CAD build for the part. Positions are in the model's coordinates, mm. A direction names the side the tool comes from. Round coordinates to 2 decimals unless told otherwise and drop trailing zeros. Write each loop counter-clockwise with the first axis right and the second up, starting at its lowest first coordinate (ties: lowest second). Pieces come first, ordered by that corner, then holes. Notation, with made-up numbers: (81.25, 22) -> (106.25, 22) arc R22 cw to (106.25, 59) -> close; hole circle Ø10 at (7.25, 16.5). An arc over 180 degrees is marked (long way). Answer in a Markdown table with one row per item. Add a question column.
Autodesk Inventor part; units mm, degrees
ref_plane "YZ Plane" through (0, 0, 0) normal (1, 0, 0) x (0, 1, 0)
ref_plane "XZ Plane" through (0, 0, 0) normal (0, 1, 0) x (-1, 0, 0)
ref_plane "XY Plane" through (0, 0, 0) normal (0, 0, 1) x (1, 0, 0)
sketch "スケッチ1" plane through (0, 0, 0) normal (0, 0, 1) x (1, 0, 0)
  line L0 (0, 0) -> (32, 0)
  line L1 (32, 0) -> (32, 32)
  line L2 (32, 32) -> (0, 32)
  line L3 (0, 32) -> (0, 0)
  dimension "d0" = 32
  dimension "d1" = 32
extrude "押し出し1" add sketch "スケッチ1" along normal blind 1.6
sketch "スケッチ2" plane through (0, 0, 1.6) normal (0, 0, 1) x (1, 0, 0)
  line L0 (0, 0) -> (32, 0)
  line L1 (32, 0) -> (32, 32)
  line L2 (32, 32) -> (0, 32)
  line L3 (0, 32) -> (0, 0)
  line L4 (30, 2) -> (2, 2)
  line L5 (2, 2) -> (2, 30)
  line L6 (2, 30) -> (30, 30)
  line L7 (30, 30) -> (30, 2)
  dimension "d4" = 28
hole "穴1" at (30, 30, 1.6) at (30, 2, 1.6) at (2, 2, 1.6) at (2, 30, 1.6) direction (0, 0, -1) diameter 2 end through all
sketch "スケッチ3" plane through (0, 0, 1.6) normal (0, 0, 1) x (1, 0, 0)
  line L0 (5.5, 26.5) -> (26.5, 26.5)
  line L1 (26.5, 26.5) -> (26.5, 5.5)
  line L2 (26.5, 5.5) -> (5.5, 5.5)
  line L3 (5.5, 5.5) -> (5.5, 26.5)
  circle A0 centre (2, 2) radius 1
  circle A1 centre (30, 30) radius 1
  circle A2 centre (30, 2) radius 1
  circle A3 centre (2, 30) radius 1
  line L4 (0, 0) -> (32, 0)
  line L5 (32, 0) -> (32, 32)
  line L6 (32, 32) -> (0, 32)
  line L7 (0, 32) -> (0, 0)
  line L8 (16, 26.5) -> (16, 32)
  line L9 (32, 32) -> (0, 32)
  line L10 (5.5, 16) -> (0, 16)
  line L11 (0, 32) -> (0, 0)
  dimension "d12" = 21
  dimension "d13" = 21
extrude "押し出し2" add sketch "スケッチ3" along normal blind 6.3 contours L0 L1 L2 L3
sketch "スケッチ4" plane through (0, 0, 7.9) normal (0, 0, 1) x (1, 0, 0)
  line L0 (5.5, 26.5) -> (5.5, 5.5)
  line L1 (5.5, 5.5) -> (26.5, 5.5)
  line L2 (26.5, 5.5) -> (26.5, 26.5)
  line L3 (26.5, 26.5) -> (5.5, 26.5)
  line L4 (5.5, 26.5) -> (26.5, 26.5)
  line L5 (16, 26.5) -> (16, 5.5)
  line L6 (5.5, 5.5) -> (26.5, 5.5)
  circle A0 centre (16, 16) radius 9.5
  point P0 (0, 0)
  dimension "d16" = 19
extrude "押し出し3" add sketch "スケッチ4" along normal blind 11.2 contours A0 L5 | L5 A0
sketch "スケッチ5" plane through (16, 16, 19.1) normal (0, 0, 1) x (1, 0, 0)
  circle A0 centre (0, 0) radius 9.5
  circle A1 centre (0, 0) radius 7
  point P0 (-16, -16)
  dimension "d19" = 14
extrude "押し出し4" add sketch "スケッチ5" along normal blind 2.5 contours A1
fillet "フィレット1" radius 7 1 edges at (9, 16, 21.6)
sketch "スケッチ6" plane through (0, 0, 0) normal (0, 0, -1) x (-1, 0, 0)
  line L0 (-14, 4.1) -> (-6, 4.1)
  line L1 (-6, 4.1) -> (-6, 0.9)
  line L2 (-6, 0.9) -> (-14, 0.9)
  line L3 (-14, 0.9) -> (-14, 4.1)
  line L4 (0, 0) -> (-32, 0)
  line L5 (0, 32) -> (0, 0)
  dimension "d23" = 8
  dimension "d24" = 3.2
  dimension "d25" = 4.1
  dimension "d26" = 14
extrude "押し出し5" add sketch "スケッチ6" along normal blind 5.5
chamfer "面取り1" distance 3 angle 45 4 edges at (5.5, 5.5, 4.75) (26.5, 5.5, 4.75) (26.5, 26.5, 4.75) (5.5, 26.5, 4.75)
properties part number "超広角カメラ_MCM-4350FISH"
Item 1: Saw through at D-D on y = 28. Give the cut face in (x, z).
Item 2: Saw through at B-B on y = 2. Give the cut face in (x, z), then the cut area to 3 significant figures.
Item 3: Pin check, flat tips, straight feed: pin 1 (10 mm diameter, centred on y = 28, z = 8.5, fed in from +X); pin 2 (4 mm diameter, centred on x = 21, y = 6.5, fed in from -Z); pin 3 (6 mm diameter, centred on x = 6.5, y = 4, fed in from +Z); pin 4 (1.2 mm diameter, centred on x = 30, y = 2, fed in from +Z). Stop position of each tip, or through.
Item 4: Saw through at C-C on z = 14.75. Give the cut face in (x, y), then the cut area to 3 significant figures.
Item 5: Two-plate mould, pull along X, no slides. Class faces 1 (the flat face through (10, 3, -5.5)), 2 (the flat face through (7, 7, 5)), 3 (the flat face through (32, 16, 1)), 4 (the cylindrical face through (2, 29, 1)): +X half, -X half, draft (parallel to the pull), parting line (faces both ways), or undercut.
Item 6: Drill centre lines: probe 1 along X at (y, z) = (30, 1.25); probe 2 along Z at (x, y) = (30, 21.5). Where is each one in solid material? Low to high.
Item 7: Saw through at A-A on x = 30. Give the cut face in (y, z), then the cut area to 3 significant figures.
Item 8: Tool access for faces 5 (the flat face through (14, 2, -3)), 6 (the flat face through (10, 0.9, -3)), 7 (the flat face through (10, 4.1, -3)), 8 (the flat face through (25, 25, 5)), 9 (the flat face through (25, 7, 5)): list every direction of +Z, -Z, +X, -X, +Y, -Y with a clear straight run to the whole face (end or side of a thin tool).
Recorded:
| question | item | result |
|---|---|---|
| 1 | outline | (0, 0) -> (32, 0) -> (32, 1.6) -> (0, 1.6) -> close |
| 2 | outline | (0, 0) -> (1, 0) -> (1, 1.6) -> (0, 1.6) -> close; (3, 0) -> (6, 0) -> (6, -5.5) -> (14, -5.5) -> (14, 0) -> (29, 0) -> (29, 1.6) -> (3, 1.6) -> close; (31, 0) -> (32, 0) -> (32, 1.6) -> (31, 1.6) -> close |
| 2 | area | 88.8 mm2 |
| 3 | pin 1 | x = 26.5 |
| 3 | pin 2 | z = 0 |
| 3 | pin 3 | z = 7.9 |
| 3 | pin 4 | through |
| 4 | outline | circle Ø19 at (16, 16) |
| 4 | area | 284 mm2 |
| 5 | face 1 | draft |
| 5 | face 2 | -X half |
| 5 | face 3 | +X half |
| 5 | face 4 | undercut |
| 6 | probe 1 | 0 to 1, 3 to 29, 31 to 32 |
| 6 | probe 2 | 0 to 1.6 |
| 7 | outline | (0, 0) -> (1, 0) -> (1, 1.6) -> (0, 1.6) -> close; (3, 0) -> (29, 0) -> (29, 1.6) -> (3, 1.6) -> close; (31, 0) -> (32, 0) -> (32, 1.6) -> (31, 1.6) -> close |
| 7 | area | 44.8 mm2 |
| 8 | face 5 | -Z, +X, +Y, -Y |
| 8 | face 6 | -Z, +X, -X, -Y |
| 8 | face 7 | -Z, +X, -X, +Y |
| 8 | face 8 | +Z, +X, +Y |
| 8 | face 9 | +Z, +X, -Y |
